from build123d import *

# Parameters (mm, degrees)
SKETCH006_W     = 36
SKETCH006_H     = 67
PAD003_DEPTH    = 2
SKETCH007_R     = 2.125
PAD004_DEPTH    = 4
SKETCH012_R     = 1.1
POCKET002_DEPTH = 2.001
SKETCH022_R     = 0.8
POCKET008_DEPTH = 6.001
SKETCH040_R     = 2.25
PAD024_DEPTH    = 20
SKETCH041_R     = 1.1303
POCKET012_DEPTH = 22.001
SKETCH047_R     = 0.8
SKETCH047_W     = 2
SKETCH047_H     = 33.5
POCKET_DEPTH    = 22.001


with BuildPart() as part:
    # Sketch006 → Pad003 (new body)
    with BuildSketch(Plane.XY):
        with Locations((18, 33.5)):
            Rectangle(SKETCH006_W, SKETCH006_H)
    extrude(amount=PAD003_DEPTH)

    # Sketch007 (on DatumPlane) → Pad004 (join)
    with BuildSketch(Plane.XY.offset(2)):
        with Locations((12.3, 57)):
            Circle(SKETCH007_R)
        with Locations((23.7, 57)):
            Circle(SKETCH007_R)
        with Locations((23.7, 10)):
            Circle(SKETCH007_R)
        with Locations((12.3, 10)):
            Circle(SKETCH007_R)
    extrude(amount=PAD004_DEPTH)

    # Sketch012 (on DatumPlane) → Pocket002 (cut, through all)
    with BuildSketch(Plane.XY.offset(2)):
        with Locations((2.2, 64.8)):
            Circle(SKETCH012_R)
        with Locations((33.8, 64.8)):
            Circle(SKETCH012_R)
        with Locations((33.8, 2.2)):
            Circle(SKETCH012_R)
        with Locations((2.2, 2.2)):
            Circle(SKETCH012_R)
        with BuildLine():
            ThreePointArc((10.11, 59), (9.11, 60), (8.11, 59))
            Line((8.11, 59), (8.11, 8))
            ThreePointArc((8.11, 8), (9.11, 7), (10.11, 8))
            Line((10.11, 8), (10.11, 59))
        make_face()
        with BuildLine():
            ThreePointArc((25.89, 8), (26.89, 7), (27.89, 8))
            Line((27.89, 8), (27.89, 59))
            ThreePointArc((27.89, 59), (26.89, 60), (25.89, 59))
            Line((25.89, 59), (25.89, 8))
        make_face()
    extrude(amount=-POCKET002_DEPTH, mode=Mode.SUBTRACT)

    # Sketch022 → Pocket008 (cut, through all)
    with BuildSketch(Plane.XY):
        with Locations((12.3, 10)):
            Circle(SKETCH022_R)
        with Locations((23.7, 10)):
            Circle(SKETCH022_R)
        with Locations((12.3, 57)):
            Circle(SKETCH022_R)
        with Locations((23.7, 57)):
            Circle(SKETCH022_R)
    extrude(amount=POCKET008_DEPTH, mode=Mode.SUBTRACT)

    # Sketch040 (on DatumPlane) → Pad024 (join)
    with BuildSketch(Plane.XY.offset(2)):
        with Locations((5.1, 9.1)):
            Circle(SKETCH040_R)
        with Locations((30.9, 9.1)):
            Circle(SKETCH040_R)
        with Locations((5.1, 38.4)):
            Circle(SKETCH040_R)
        with Locations((30.9, 38.4)):
            Circle(SKETCH040_R)
    extrude(amount=PAD024_DEPTH)

    # Sketch041 → Pocket012 (cut, through all)
    with BuildSketch(Plane.XY):
        with Locations((5.1, 38.4)):
            Circle(SKETCH041_R)
        with Locations((30.9, 38.4)):
            Circle(SKETCH041_R)
        with Locations((30.9, 9.1)):
            Circle(SKETCH041_R)
        with Locations((5.1, 9.1)):
            Circle(SKETCH041_R)
    extrude(amount=POCKET012_DEPTH, mode=Mode.SUBTRACT)

    # Sketch047 → Pocket (cut, through all)
    with BuildSketch(Plane.XY):
        with Locations((18, 2.2)):
            Circle(SKETCH047_R)
        with Locations((9.11, 16.75)):
            Rectangle(SKETCH047_W, SKETCH047_H)
        with Locations((26.89, 16.75)):
            Rectangle(SKETCH047_W, SKETCH047_H)
    extrude(amount=POCKET_DEPTH, mode=Mode.SUBTRACT)


with BuildPart() as part_1:
    # Body002 placement: moved
    add(part.part.moved(Location((0, 0, 15.75))))


solid = part_1.part
Verification items for the finished model (mm, model axes). A direction names the side the tool comes from. Give positions to 0.01 mm unless a question says otherwise; leave off trailing zeros. Write each loop counter-clockwise with the first axis right and the second up, starting at its lowest first coordinate (ties: lowest second). Pieces come first, ordered by that corner, then holes.
(1) Access from +Z, -Z, +X, -X, +Y, -Y to the whole of each face (thin tool, end or side, straight path). Record for faces 1 (the face through (4, 10, 37.75)), 2 (the face through (22.1, 58.4, 19.7)), 3 (the face through (10.11, 29, 17)).
(2) Material ranges on line 1 (Y direction, x = 5, z = 28); line 2 (Y direction, x = 23.7, z = 18) (3 decimals); line 3 (Z direction, x = 34, y = 46.5), recorded low to high.
(3) Cross-section at B-B (y = 57). Enter the section's corners in (x, z) (3 decimals).
(4) Mould release check, pull along X, two halves, no side actions. Record for faces 4 (the face through (1.962, 1.126, 16.764)), 5 (the face through (6, 37, 37.75)), 6 (the face through (10.61, 8.71, 19.72)): +X half, -X half, draft (parallel to the pull), parting line (faces both ways), or undercut.
(5) Gauge pin test, flat ends, axial feed: pin 1 (0.6 mm diameter, centred on y = 37.5, z = 16.5, fed in from -X); pin 2 (3 mm diameter, centred on y = 11, z = 34.5, fed in from -X); pin 3 (5 mm diameter, centred on x = 5, z = 28.5, fed in from -Y); pin 4 (11 mm diameter, centred on x = 25, y = 22, fed in from +Z). Record the tip position at first contact, or that the pin passes through.
(6) Cross-section at D-D (y = 21). Enter the section's corners in (x, z).
(7) Cross-section at C-C (x = 5.1). Enter the section's corners in (y, z).
(8) Cross-section at A-A (z = 25.5). Enter the section's corners in (x, y), plus the area to 3 significant figures.
Worked out:
1. face 1: +Z, +X, -X, +Y, -Y
1. face 2: +Z
1. face 3: +Z, -Z, -Y
2. line 1: y = 6.85 to 7.97, 10.23 to 11.35, 36.15 to 37.27, 39.53 to 40.65
2. line 2: y = 7.875 to 9.2, 10.8 to 12.125, 54.875 to 56.2, 57.8 to 59.125
2. line 3: z = 15.75 to 17.75
3. outline: (0, 15.75) - (8.11, 15.75) - (8.11, 17.75) - (0, 17.75) - close; (10.11, 15.75) - (11.5, 15.75) - (11.5, 21.75) - (10.175, 21.75) - (10.175, 17.75) - (10.11, 17.75) - close; (13.1, 15.75) - (22.9, 15.75) - (22.9, 21.75) - (21.575, 21.75) - (21.575, 17.75) - (14.425, 17.75) - (14.425, 21.75) - (13.1, 21.75) - close; (24.5, 15.75) - (25.89, 15.75) - (25.89, 17.75) - (25.825, 17.75) - (25.825, 21.75) - (24.5, 21.75) - close; (27.89, 15.75) - (36, 15.75) - (36, 17.75) - (27.89, 17.75) - close
4. face 4: undercut
4. face 5: draft
4. face 6: undercut
5. pin 1: stops at x = 0
5. pin 2: stops at x = 2.89
5. pin 3: stops at y = 6.85
5. pin 4: stops at z = 17.75
6. outline: (0, 15.75) - (8.11, 15.75) - (8.11, 17.75) - (0, 17.75) - close; (10.11, 15.75) - (25.89, 15.75) - (25.89, 17.75) - (10.11, 17.75) - close; (27.89, 15.75) - (36, 15.75) - (36, 17.75) - (27.89, 17.75) - close
7. outline: (0, 15.75) - (7.97, 15.75) - (7.97, 37.75) - (6.85, 37.75) - (6.85, 17.75) - (0, 17.75) - close; (10.23, 15.75) - (37.27, 15.75) - (37.27, 37.75) - (36.15, 37.75) - (36.15, 17.75) - (11.35, 17.75) - (11.35, 37.75) - (10.23, 37.75) - close; (39.53, 15.75) - (67, 15.75) - (67, 17.75) - (40.65, 17.75) - (40.65, 37.75) - (39.53, 37.75) - close
8. outline: circle Ø4.5 at (5.1, 9.1); circle Ø4.5 at (5.1, 38.4); circle Ø4.5 at (30.9, 9.1); circle Ø4.5 at (30.9, 38.4); hole circle Ø2.26 at (5.1, 9.1); hole circle Ø2.26 at (5.1, 38.4); hole circle Ø2.26 at (30.9, 9.1); hole circle Ø2.26 at (30.9, 38.4)
8. area: 47.6 mm2
